```python
from build123d import *

# Parameters (mm, degrees)
SKETCH_W        = 116
SKETCH_H        = 190
PAD_DEPTH       = 38
SKETCH001_W     = 113.6
SKETCH001_H     = 187.6
POCKET_DEPTH    = 36.6
SKETCH037_R     = 1.25
POCKET007_DEPTH = 38.001
SKETCH002_R     = 3.5
SKETCH002_R_2   = 1
PAD031_DEPTH    = 2.5
SKETCH036_R     = 3.5
PAD032_DEPTH    = 2.2
SKETCH053_R     = 1.15
POCKET016_DEPTH = 3
POCKET017_DEPTH = 1.4


with BuildPart() as part:
    # Sketch → Pad (new body)
    with BuildSketch(Plane.XY):
        Rectangle(SKETCH_W, SKETCH_H)
    extrude(amount=PAD_DEPTH)

    # Sketch001 (on DatumPlane) → Pocket (cut)
    with BuildSketch(Plane.XY.offset(38)):
        Rectangle(SKETCH001_W, SKETCH001_H)
    extrude(amount=-POCKET_DEPTH, mode=Mode.SUBTRACT)

    # Sketch037 → Pocket007 (cut, through all)
    with BuildSketch(Plane(origin=(0, 0, 0), x_dir=(1, 0, 0), z_dir=(0, 0, -1))):
        with Locations((33.2, 2)):
            Circle(SKETCH037_R)
        with Locations((-33.2, 2)):
            Circle(SKETCH037_R)
        with Locations((33.2, 47)):
            Circle(SKETCH037_R)
        with Locations((-33.2, 47)):
            Circle(SKETCH037_R)
    extrude(amount=-POCKET007_DEPTH, mode=Mode.SUBTRACT)

    # Sketch002 (on Face15 of Pocket007) → Pad031 (join)
    with BuildSketch(Plane.XY.offset(1.4)):
        with Locations((12.249996, 81.49999)):
            Circle(SKETCH002_R)
        with Locations((12.249996, 81.49999)):
            Circle(SKETCH002_R_2, mode=Mode.SUBTRACT)
        with Locations((12.249996, 53.49999)):
            Circle(SKETCH002_R)
        with Locations((12.249996, 53.49999)):
            Circle(SKETCH002_R_2, mode=Mode.SUBTRACT)
        with Locations((-23.250004, 67.49999)):
            Circle(SKETCH002_R)
        with Locations((-23.250004, 67.49999)):
            Circle(SKETCH002_R_2, mode=Mode.SUBTRACT)
        with Locations((30.749948, 59.999954)):
            Circle(SKETCH002_R)
        with Locations((30.749948, 59.999954)):
            Circle(SKETCH002_R_2, mode=Mode.SUBTRACT)
        with Locations((44.749948, 24.499954)):
            Circle(SKETCH002_R)
        with Locations((44.749948, 24.499954)):
            Circle(SKETCH002_R_2, mode=Mode.SUBTRACT)
        with Locations((16.749948, 24.499954)):
            Circle(SKETCH002_R)
        with Locations((16.749948, 24.499954)):
            Circle(SKETCH002_R_2, mode=Mode.SUBTRACT)
        with Locations((30.749994, -13.50001)):
            Circle(SKETCH002_R)
        with Locations((30.749994, -13.50001)):
            Circle(SKETCH002_R_2, mode=Mode.SUBTRACT)
        with Locations((44.749994, -49.00001)):
            Circle(SKETCH002_R)
        with Locations((44.749994, -49.00001)):
            Circle(SKETCH002_R_2, mode=Mode.SUBTRACT)
        with Locations((16.749994, -49.00001)):
            Circle(SKETCH002_R)
        with Locations((16.749994, -49.00001)):
            Circle(SKETCH002_R_2, mode=Mode.SUBTRACT)
        with Locations((22.749996, -67.500006)):
            Circle(SKETCH002_R)
        with Locations((22.749996, -67.500006)):
            Circle(SKETCH002_R_2, mode=Mode.SUBTRACT)
        with Locations((-12.750004, -53.500006)):
            Circle(SKETCH002_R)
        with Locations((-12.750004, -53.500006)):
            Circle(SKETCH002_R_2, mode=Mode.SUBTRACT)
        with Locations((-12.750004, -81.500006)):
            Circle(SKETCH002_R)
        with Locations((-12.750004, -81.500006)):
            Circle(SKETCH002_R_2, mode=Mode.SUBTRACT)
        with Locations((-31.249992, -60.000005)):
            Circle(SKETCH002_R)
        with Locations((-31.249992, -60.000005)):
            Circle(SKETCH002_R_2, mode=Mode.SUBTRACT)
        with Locations((-45.249992, -24.500005)):
            Circle(SKETCH002_R)
        with Locations((-45.249992, -24.500005)):
            Circle(SKETCH002_R_2, mode=Mode.SUBTRACT)
        with Locations((-17.249992, -24.500005)):
            Circle(SKETCH002_R)
        with Locations((-17.249992, -24.500005)):
            Circle(SKETCH002_R_2, mode=Mode.SUBTRACT)
        with Locations((-44.749987, 48.499969)):
            Circle(SKETCH002_R)
        with Locations((-44.749987, 48.499969)):
            Circle(SKETCH002_R_2, mode=Mode.SUBTRACT)
        with Locations((-16.749987, 48.499969)):
            Circle(SKETCH002_R)
        with Locations((-16.749987, 48.499969)):
            Circle(SKETCH002_R_2, mode=Mode.SUBTRACT)
        with Locations((-30.749987, 12.999969)):
            Circle(SKETCH002_R)
        with Locations((-30.749987, 12.999969)):
            Circle(SKETCH002_R_2, mode=Mode.SUBTRACT)
        with Locations((12.249996, 8.49999)):
            Circle(SKETCH002_R)
        with Locations((12.249996, 8.49999)):
            Circle(SKETCH002_R_2, mode=Mode.SUBTRACT)
        with Locations((12.249996, -19.50001)):
            Circle(SKETCH002_R)
        with Locations((12.249996, -19.50001)):
            Circle(SKETCH002_R_2, mode=Mode.SUBTRACT)
        with Locations((-23.250004, -5.50001)):
            Circle(SKETCH002_R)
        with Locations((-23.250004, -5.50001)):
            Circle(SKETCH002_R_2, mode=Mode.SUBTRACT)
    extrude(amount=PAD031_DEPTH)

    # Sketch036 (on Face15 of Pad031) → Pad032 (join)
    with BuildSketch(Plane.XY.offset(1.4)):
        with Locations((33.2, -2)):
            Circle(SKETCH036_R)
        with Locations((-33.2, -2)):
            Circle(SKETCH036_R)
        with Locations((33.2, -47)):
            Circle(SKETCH036_R)
        with Locations((-33.2, -47)):
            Circle(SKETCH036_R)
    extrude(amount=PAD032_DEPTH)

    # Sketch053 (on Face4 of Pad032) → Pocket016 (cut)
    with BuildSketch(Plane(origin=(0, 0, 0), x_dir=(1, 0, 0), z_dir=(0, 0, -1))):
        with Locations((-33.2, 47)):
            Circle(SKETCH053_R)
        with Locations((33.2, 47)):
            Circle(SKETCH053_R)
        with Locations((33.2, 2)):
            Circle(SKETCH053_R)
        with Locations((-33.2, 2)):
            Circle(SKETCH053_R)
    extrude(amount=-POCKET016_DEPTH, mode=Mode.SUBTRACT)

    # Sketch076 (on Face19 of Pocket016) → Pocket017 (cut)
    with BuildSketch(Plane.XY.offset(1.4)):
        Polygon((-51.224859, 22.025095), (-44.507345, 15.30758), (-42.032471, 17.782454), (-48.749985, 24.499969), align=None)
        Polygon((-51.724864, -50.974879), (-45.00735, -57.692393), (-42.53246, -55.217536), (-49.24999, -48.500005), align=None)
        Polygon((11.249996, -85.500006), (17.96751, -78.782491), (20.442384, -81.257365), (13.724869, -87.974879), align=None)
        Polygon((42.032481, -18.282496), (48.749995, -25.00001), (51.224869, -22.525137), (44.507354, -15.807622), align=None)
        Polygon((42.032435, 55.217468), (48.749949, 48.499953), (51.224823, 50.974827), (44.507309, 57.692341), align=None)
        Polygon((-19.531949, 7.051014), (-11.750004, 12.49999), (-13.757522, 15.367023), (-21.539466, 9.918046), align=None)
        Polygon((-18.467519, 76.782476), (-11.750004, 83.49999), (-14.224878, 85.974864), (-20.942392, 79.25735), align=None)
    extrude(amount=-POCKET017_DEPTH, mode=Mode.SUBTRACT)


with BuildPart() as part_1:
    # Body placement: moved
    add(part.part.moved(Location((0, 5, 0))))


solid = part_1.part
```
The listing builds one solid part. Answer for the finished solid, in the listing's coordinates (mm). A direction names the side the tool comes from. Give positions to 0.01 mm unless a question says otherwise; leave off trailing zeros. Order: outer loops, then holes, each group sorted by start corner. A loop starts at its lowest first (then second) coordinate and runs counter-clockwise, first axis right, second up. Notation, with made-up numbers: (48.25, 40.5) -> (93.25, 40.5) arc R21 cw to (93.25, 46.5) -> close; hole circle Ø9 at (50, 69.5). An arc over 180 degrees is marked (long way). One line per item, written item: value.
1) Determine the mould class of faces 3 (the flat face through (58, 4, 19)), 4 (the cylindrical face through (-17.71, -16.03, 2.63)) for opening direction Y: pulls with the +Y half, pulls with the -Y half, needs draft (parallel to the pull), parting line crosses it, or undercut.
Reported:
face 3: needs draft
face 4: undercut
2) Find section B-B, the plane z = 9.5. Determine the outline of the cut face in (x, y), plus the area to 3 significant figures.
Reported:
outline: (-58, -90) -> (58, -90) -> (58, 100) -> (-58, 100) -> close; hole (-56.8, -88.8) -> (56.8, -88.8) -> (56.8, 98.8) -> (-56.8, 98.8) -> close
area: 729 mm^2
3) Flat-ended cylindrical pins translate along their axes: P1, Ø0.6, axis at x = 12.5, y = 58, coming from the +Z side; P2, Ø2, axis at x = -33, y = -42, coming from the -Z side; P3, Ø3, axis at x = 36, y = 37.5, coming from the -Z side; P4, Ø7.5, axis at x = 12, y = 86, coming from the +Z side. Find the tip coordinate at first contact, or state that the pin passes through.
Reported:
P1: stops at z = 1.4
P2: stops at z = 1.4
P3: stops at z = 0
P4: stops at z = 3.9
4) A tool of negligible diameter and unlimited length cuts with its end or side. For faces 1 (the flat face through (-15.695, 14.737, 0.71)), 2 (the flat face through (11, 58, 3.9)), from which of +Z, -Z, +X, -X, +Y, -Y can it reach the whole face along a straight path? Write none if from no direction.
Reported:
face 1: +Z, -Z
face 2: +Z
5) Find the intervals of material crossed by line 1 (Y direction, x = 41, z = 30.5); line 2 (X direction, y = 26, z = 24); line 3 (X direction, y = -53, z = 2), in increasing order.
Reported:
line 1: y = -90 to -88.8, 98.8 to 100
line 2: x = -58 to -56.8, 56.8 to 58
line 3: x = -58 to -56.8, -34.12 to -28.38, 56.8 to 58
6) Find section A-A, the plane y = 42.5. Determine the outline of the cut face in (x, z).
Reported:
outline: (-58, 0) -> (58, 0) -> (58, 38) -> (56.8, 38) -> (56.8, 1.4) -> (-56.8, 1.4) -> (-56.8, 38) -> (-58, 38) -> close
